Autodesk Inventor part; units mm, degrees
ref_plane "YZ Plane" through (0, 0, 0) normal (1, 0, 0) x (0, 1, 0)
ref_plane "XZ Plane" through (0, 0, 0) normal (0, 1, 0) x (-1, 0, 0)
ref_plane "XY Plane" through (0, 0, 0) normal (0, 0, 1) x (1, 0, 0)
sketch "スケッチ1" plane through (0, 0, 0) normal (0, 1, 0) x (-1, 0, 0)
  line L0 (0, 0) -> (-81.5097, 0)
  line L1 (-81.5097, 0) -> (-81.5097, -169)
  line L2 (-81.5097, -169) -> (0, -169)
  line L3 (0, -169) -> (0, 0)
  dimension "d0" = 169
  dimension "d7" = 81.5097
extrude "押し出し1" add sketch "スケッチ1" along normal blind 2
fillet "フィレット1" radius 4.5 4 edges at (81.5097, 1, 0) (0, 1, 0) (81.5097, 1, -169) (0, 1, -169)
sketch "スケッチ3" plane through (0, 0, 0) normal (0, -1, 0) x (1, 0, 0)
  line L0 (81.5097, -4.5) -> (81.5097, -164.5)
  line L1 (0, -164.5) -> (0, -4.5)
  line L2 (77.0097, -169) -> (4.5, -169)
  line L3 (4.5, 0) -> (77.0097, 0)
  point P0 (0, 0)
  point P1 (77.0097, -4.5)
  point P2 (77.0097, -164.5)
  point P3 (4.5, -164.5)
  point P4 (4.5, -4.5)
  dimension "d34" = 4.5
  dimension "d35" = 4.5
  dimension "d36" = 4.5
  dimension "d37" = 4.5
  dimension "d38" = 4.5
  dimension "d39" = 4.5
  dimension "d40" = 4.5
  dimension "d41" = 4.5
hole "穴2" at (77.0097, 0, -4.5) at (77.0097, 0, -164.5) at (4.5, 0, -164.5) at (4.5, 0, -4.5) direction (0, 1, 0) diameter 3 end through all
sketch "スケッチ4" plane through (0, 0, 0) normal (0, -1, 0) x (1, 0, 0)
  line L0 (66.5097, -73) -> (17.5097, -73)
  line L1 (17.5097, -73) -> (17.5097, -15)
  line L2 (17.5097, -15) -> (66.5097, -15)
  line L3 (66.5097, -15) -> (66.5097, -73)
  line L4 (81.5097, -4.5) -> (81.5097, -164.5)
  line L5 (4.5, 0) -> (77.0097, 0)
  point P0 (0, 0)
  dimension "d49" = 49
  dimension "d50" = 58
  dimension "d51" = 15
  dimension "d52" = 15
hole "穴3" at (66.5097, 0, -73) at (17.5097, 0, -73) at (17.5097, 0, -15) at (66.5097, 0, -15) direction (0, 1, 0) diameter 3 end through all
ref_plane "作業平面1" through (81.5097, 2, 0) normal (-1, 0, 0) x (0, 0, -1)
properties part number "ロボット回転_回路ボード1_CPY" material "木材 (カエデ材)"
Model file for the job. Use its own axes, mm. Coordinates: 2 decimals unless noted, no trailing zeros. Return JSON: item names as keys, results as strings.
1. Drill centre lines: probe 1 along X at (y, z) = (0.85, -15); probe 2 along Z at (x, y) = (17.5, 1.3); probe 3 along X at (y, z) = (1.45, -164.5). Where is each one in solid material? Low to high.
Ans:
{"probe 1": "0 to 16.01, 19.01 to 65.01, 68.01 to 81.51", "probe 2": "-169 to -74.5, -71.5 to -16.5, -13.5 to 0", "probe 3": "0 to 3, 6 to 75.51, 78.51 to 81.51"}
2. Pull direction X, two halves, no side cores. Call faces 1 (the face through (41, 0, -83)), 2 (the face through (78.34, 1.01, -5.19)), 3 (the face through (1.283, 1.014, -1.353)): +X half, -X half, draft (parallel to the pull), parting line (faces both ways), or undercut.
Ans:
{"face 1": "draft", "face 2": "undercut", "face 3": "-X half"}
3. Flat gauge pin, fed straight in: pin 1 (2.5 mm diameter, centred on x = 66.51, z = -15, fed in from +Y). Where does the tip first touch, or does it go through?
Ans:
{"pin 1": "through"}
